Geometry check sheet. Reference: the model listing, model coordinates, mm. Coordinates: 2 decimals unless noted, no trailing zeros. Write each loop counter-clockwise with the first axis right and the second up, starting at its lowest first coordinate (ties: lowest second). Pieces come first, ordered by that corner, then holes. Notation, with made-up numbers: (35.5, -21) -> (50.5, -21) arc R24 cw to (50.5, -8) -> close; hole circle Ø10 at (64, -25.5). An arc over 180 degrees is marked (long way). One line per question, with ' | ' between items.
from build123d import *

# Parameters (mm, degrees)
EXTRUDE_1_DEPTH     = 3
SKETCH_2_R          = 1.5
CUT_EXTRUDE_1_DEPTH = 3
CUT_EXTRUDE_2_DEPTH = 10
SKETCH_4_R          = 1.5
CUT_EXTRUDE_3_DEPTH = 4
SKETCH_5_R          = 1.5
CUT_EXTRUDE_4_DEPTH = 10
SKETCH_6_R          = 1.5
CUT_EXTRUDE_5_DEPTH = 10


with BuildPart() as part:
    # 草图1 → 凸台-拉伸1 (new body)
    with BuildSketch(Plane(origin=(0, 0, 0), x_dir=(1, 0, 0), z_dir=(0, 1, 0))):
        with BuildLine():
            Line((-108.354700855, 61.431623932), (81.645299145, 61.431623932))
            ThreePointArc((81.645299145, 61.431623932), (102.858502581, 52.644827367), (111.645299145, 31.431623932))
            Line((111.645299145, 31.431623932), (111.645299145, -33.568376068))
            ThreePointArc((111.645299145, -33.568376068), (102.858502581, -54.781579504), (81.645299145, -63.568376068))
            Line((81.645299145, -63.568376068), (-108.354700855, -63.568376068))
            ThreePointArc((-108.354700855, -63.568376068), (-129.56790429, -54.781579504), (-138.354700855, -33.568376068))
            Line((-138.354700855, -33.568376068), (-138.354700855, 31.431623932))
            ThreePointArc((-138.354700855, 31.431623932), (-129.56790429, 52.644827367), (-108.354700855, 61.431623932))
        make_face()
    extrude(amount=EXTRUDE_1_DEPTH)

    # 草图2 → 切除-拉伸1 (cut)
    with BuildSketch(Plane(origin=(0, 3, 0), x_dir=(1, 0, 0), z_dir=(0, 1, 0))):
        with Locations((-78.354700855, -45.568376068)):
            Circle(SKETCH_2_R)
        with Locations((-78.354700855, -57.568376068)):
            Circle(SKETCH_2_R)
        with Locations((51.645299145, -45.568376068)):
            Circle(SKETCH_2_R)
        with Locations((51.645299145, -57.568376068)):
            Circle(SKETCH_2_R)
        with Locations((-78.354700855, 55.431623932)):
            Circle(SKETCH_2_R)
        with Locations((-78.354700855, 43.431623932)):
            Circle(SKETCH_2_R)
        with Locations((51.645299145, 43.431623932)):
            Circle(SKETCH_2_R)
        with Locations((51.645299145, 55.431623932)):
            Circle(SKETCH_2_R)
    extrude(amount=-CUT_EXTRUDE_1_DEPTH, mode=Mode.SUBTRACT)

    # 草图3 → 切除-拉伸2 (cut)
    with BuildSketch(Plane(origin=(0, 3, 0), x_dir=(1, 0, 0), z_dir=(0, 1, 0))):
        with BuildLine():
            Line((-127.854700855, -30), (-127.854700855, 30))
            ThreePointArc((-127.854700855, 30), (-126.354700855, 31.5), (-124.854700855, 30))
            Line((-124.854700855, 30), (-124.854700855, -30))
            ThreePointArc((-124.854700855, -30), (-126.354700855, -31.5), (-127.854700855, -30))
        make_face()
        with BuildLine():
            Line((98.145299145, -30), (98.145299145, 30))
            ThreePointArc((98.145299145, 30), (99.645299145, 31.5), (101.145299145, 30))
            Line((101.145299145, 30), (101.145299145, -30))
            ThreePointArc((101.145299145, -30), (99.645299145, -31.5), (98.145299145, -30))
        make_face()
        with BuildLine():
            Line((-114.900254633, -48.02282229), (-106.12832787, -39.250895528))
            ThreePointArc((-106.12832787, -39.250895528), (-105.037220314, -39.250895528), (-105.037220314, -40.342003084))
            Line((-105.037220314, -40.342003084), (-113.809147077, -49.113929846))
            ThreePointArc((-113.809147077, -49.113929846), (-114.900254633, -49.113929846), (-114.900254633, -48.02282229))
        make_face()
        with BuildLine():
            Line((-106.195945183, -37.953473922), (-114.967871946, -29.181547159))
            ThreePointArc((-114.967871946, -29.181547159), (-114.967871946, -27.955204977), (-113.741529764, -27.955204977))
            Line((-113.741529764, -27.955204977), (-104.969603001, -36.72713174))
            ThreePointArc((-104.969603001, -36.72713174), (-104.969603001, -37.953473922), (-106.195945183, -37.953473922))
        make_face()
        with BuildLine():
            Line((-102.683942112, -39.353763801), (-93.91201535, -48.125690563))
            ThreePointArc((-93.91201535, -48.125690563), (-93.91201535, -49.011061573), (-94.79738636, -49.011061573))
            Line((-94.79738636, -49.011061573), (-103.569313122, -40.239134811))
            ThreePointArc((-103.569313122, -40.239134811), (-103.569313122, -39.353763801), (-102.683942112, -39.353763801))
        make_face()
        with BuildLine():
            Line((-104.217158252, -37.476114378), (-94.832060398, -28.091016525))
            ThreePointArc((-94.832060398, -28.091016525), (-93.877341311, -28.091016525), (-93.877341311, -29.045735612))
            Line((-93.877341311, -29.045735612), (-103.262439165, -38.430833465))
            ThreePointArc((-103.262439165, -38.430833465), (-104.217158252, -38.430833465), (-104.217158252, -37.476114378))
        make_face()
        with BuildLine():
            Line((-115.372891691, 27.449814768), (-107.214136019, 35.60857044))
            ThreePointArc((-107.214136019, 35.60857044), (-105.177754347, 35.60857044), (-105.177754347, 33.572188767))
            Line((-105.177754347, 33.572188767), (-113.336510018, 25.413433095))
            ThreePointArc((-113.336510018, 25.413433095), (-115.372891691, 25.413433095), (-115.372891691, 27.449814768))
        make_face()
        with BuildLine():
            Line((-107.107809328, 37.361004116), (-115.266564999, 45.519759787))
            ThreePointArc((-115.266564999, 45.519759787), (-115.266564999, 47.343488076), (-113.44283671, 47.343488076))
            Line((-113.44283671, 47.343488076), (-105.284081039, 39.184732404))
            ThreePointArc((-105.284081039, 39.184732404), (-105.284081039, 37.361004116), (-107.107809328, 37.361004116))
        make_face()
        with BuildLine():
            Line((-103.88351943, 38.361678912), (-95.084137633, 47.16106071))
            ThreePointArc((-95.084137633, 47.16106071), (-93.625264077, 47.16106071), (-93.625264077, 45.702187154))
            Line((-93.625264077, 45.702187154), (-102.424645874, 36.902805357))
            ThreePointArc((-102.424645874, 36.902805357), (-103.88351943, 36.902805357), (-103.88351943, 38.361678912))
        make_face()
        with BuildLine():
            Line((-101.717094005, 35.386742124), (-93.558338334, 27.227986453))
            ThreePointArc((-93.558338334, 27.227986453), (-93.558338334, 25.635261411), (-95.151063376, 25.635261411))
            Line((-95.151063376, 25.635261411), (-103.309819047, 33.794017082))
            ThreePointArc((-103.309819047, 33.794017082), (-103.309819047, 35.386742124), (-101.717094005, 35.386742124))
        make_face()
        with BuildLine():
            Line((67.051420942, -47.974497865), (75.823347705, -39.202571103))
            ThreePointArc((75.823347705, -39.202571103), (77.011104111, -39.202571103), (77.011104111, -40.390327509))
            Line((77.011104111, -40.390327509), (68.239177348, -49.162254271))
            ThreePointArc((68.239177348, -49.162254271), (67.051420942, -49.162254271), (67.051420942, -47.974497865))
        make_face()
        with BuildLine():
            Line((76.026361578, -38.002790255), (67.118623268, -29.095051945))
            ThreePointArc((67.118623268, -29.095051945), (67.118623268, -28.041700191), (68.171975022, -28.041700191))
            Line((68.171975022, -28.041700191), (77.079713332, -36.949438501))
            ThreePointArc((77.079713332, -36.949438501), (77.079713332, -38.002790255), (76.026361578, -38.002790255))
        make_face()
        with BuildLine():
            Line((79.555520355, -39.114301334), (88.327447117, -47.886228097))
            ThreePointArc((88.327447117, -47.886228097), (88.327447117, -49.25052404), (86.963151173, -49.25052404))
            Line((86.963151173, -49.25052404), (78.191224411, -40.478597278))
            ThreePointArc((78.191224411, -40.478597278), (78.191224411, -39.114301334), (79.555520355, -39.114301334))
        make_face()
        with BuildLine():
            Line((78.357230227, -36.824160675), (87.12915699, -28.052233913))
            ThreePointArc((87.12915699, -28.052233913), (88.161441301, -28.052233913), (88.161441301, -29.084518224))
            Line((88.161441301, -29.084518224), (79.389514538, -37.856444987))
            ThreePointArc((79.389514538, -37.856444987), (78.357230227, -37.856444987), (78.357230227, -36.824160675))
        make_face()
        with BuildLine():
            Line((67.041358523, 27.035564554), (75.949096833, 35.943302864))
            ThreePointArc((75.949096833, 35.943302864), (77.156978077, 35.943302864), (77.156978077, 34.73542162))
            Line((77.156978077, 34.73542162), (68.249239767, 25.82768331))
            ThreePointArc((68.249239767, 25.82768331), (67.041358523, 25.82768331), (67.041358523, 27.035564554))
        make_face()
        with BuildLine():
            Line((76.086975669, 37.057823836), (67.179237359, 45.965562146))
            ThreePointArc((67.179237359, 45.965562146), (67.179237359, 46.897685718), (68.111360931, 46.897685718))
            Line((68.111360931, 46.897685718), (77.019099241, 37.989947408))
            ThreePointArc((77.019099241, 37.989947408), (77.019099241, 37.057823836), (76.086975669, 37.057823836))
        make_face()
        with BuildLine():
            Line((79.385756077, 35.987557483), (88.293494387, 27.079819173))
            ThreePointArc((88.293494387, 27.079819173), (88.293494387, 25.78342869), (86.997103904, 25.78342869))
            Line((86.997103904, 25.78342869), (78.089365594, 34.691167))
            ThreePointArc((78.089365594, 34.691167), (78.089365594, 35.987557483), (79.385756077, 35.987557483))
        make_face()
        with BuildLine():
            Line((78.097193522, 38.164252935), (87.004931832, 47.071991245))
            ThreePointArc((87.004931832, 47.071991245), (88.285666458, 47.071991245), (88.285666458, 45.791256619))
            Line((88.285666458, 45.791256619), (79.377928148, 36.883518309))
            ThreePointArc((79.377928148, 36.883518309), (78.097193522, 36.883518309), (78.097193522, 38.164252935))
        make_face()
    extrude(amount=-CUT_EXTRUDE_2_DEPTH, mode=Mode.SUBTRACT)

    # 草图4 → 切除-拉伸3 (cut, through all)
    with BuildSketch(Plane(origin=(0, 3, 0), x_dir=(1, 0, 0), z_dir=(0, 1, 0))):
        with Locations((93.645299145, -55)):
            Circle(SKETCH_4_R)
        with Locations((93.645299145, 55)):
            Circle(SKETCH_4_R)
        with Locations((-120.354700855, 55)):
            Circle(SKETCH_4_R)
        with Locations((-120.354700855, -55)):
            Circle(SKETCH_4_R)
    extrude(amount=-CUT_EXTRUDE_3_DEPTH, mode=Mode.SUBTRACT)

    # 草图5 → 切除-拉伸4 (cut)
    with BuildSketch(Plane.XZ):
        with Locations((-13.354700855, 55)):
            Circle(SKETCH_5_R)
        with Locations((-13.354700855, -55)):
            Circle(SKETCH_5_R)
    extrude(amount=-CUT_EXTRUDE_4_DEPTH, mode=Mode.SUBTRACT)

    # 草图6 → 切除-拉伸5 (cut)
    with BuildSketch(Plane(origin=(0, 3, 0), x_dir=(1, 0, 0), z_dir=(0, 1, 0))):
        with Locations((15.645299145, 55.431623932)):
            Circle(SKETCH_6_R)
        with Locations((15.645299145, 43.431623932)):
            Circle(SKETCH_6_R)
        with Locations((15.645299145, -45.568376068)):
            Circle(SKETCH_6_R)
        with Locations((15.645299145, -57.568376068)):
            Circle(SKETCH_6_R)
        with Locations((-42.354700855, -45.568376068)):
            Circle(SKETCH_6_R)
        with Locations((-42.354700855, -57.568376068)):
            Circle(SKETCH_6_R)
        with Locations((-42.354700855, 55.431623932)):
            Circle(SKETCH_6_R)
        with Locations((-42.354700855, 43.431623932)):
            Circle(SKETCH_6_R)
    extrude(amount=-CUT_EXTRUDE_5_DEPTH, mode=Mode.SUBTRACT)


solid = part.part
1. Cross-section at C-C on y = 1. Give the number of separate pieces and of enclosed holes in the cut face, and give its area (4 significant figures).
Worked answers:
separate pieces: 1 | enclosed holes: 40 | area: 29,550 mm²
2. Material ranges on line 1 (X direction, y = 0.2, z = 19); line 2 (Z direction, x = -41.5, y = 2.75); line 3 (X direction, y = 0.8, z = 36), recorded low to high. Write a range as from..to.
Worked answers:
line 1: -138.35..-127.85, -124.85..98.15, 101.15..111.65 | line 2: -61.43..-56.66, -54.2..-44.66, -42.2..44.34, 46.8..56.34, 58.8..63.57 | line 3: -138.26..-108.15, -105.7..-102.74, -100.83..74.02, 76.13..79.18, 81.25..111.55
3. Mould release check, pull along X, two halves, no side actions. Record for faces 1 (the face through (-97.963, 1.521, -41.364)), 2 (the face through (-99.545, 1.521, -42.7)), 3 (the face through (-129.333, 1.479, 55.014)): released by +X, released by -X, zero draft, split by the parting line, or undercut.
Worked answers:
face 1: undercut | face 2: undercut | face 3: released by -X
4. Cross-section at B-B on x = -98. Record the boundary of the cut face in (y, z), and give its area (3 significant figures).
Worked answers:
outline: (0, -61.43) -> (3, -61.43) -> (3, -44.25) -> (0, -44.25) -> close; (0, -41.33) -> (3, -41.33) -> (3, -31.67) -> (0, -31.67) -> close; (0, -28.48) -> (3, -28.48) -> (3, 31.26) -> (0, 31.26) -> close; (0, 33.17) -> (3, 33.17) -> (3, 44.04) -> (0, 44.04) -> close; (0, 45.81) -> (3, 45.81) -> (3, 63.57) -> (0, 63.57) -> close | area: 346 mm²
5. Cross-section at A-A on z = -16. Record the boundary of the cut face in (x, y).
Worked answers:
outline: (-138.35, 0) -> (-127.85, 0) -> (-127.85, 3) -> (-138.35, 3) -> close; (-124.85, 0) -> (98.15, 0) -> (98.15, 3) -> (-124.85, 3) -> close; (101.15, 0) -> (111.65, 0) -> (111.65, 3) -> (101.15, 3) -> close
6. Go/stop test with a flat-tipped pin: P1, Ø1.8, axis at x = 15.65, z = 57.57, coming from the -Y side. Record where the tip stops, or that it passes through.
Worked answers:
P1: through
